```python
from build123d import *

# Parameters (mm, degrees)
SKETCH1_W               = 171.8
SKETCH1_H               = 57.8
MAIN_BODY_DEPTH         = 10
SKETCH2_W               = 163.8
SKETCH2_H               = 49.8
MAIN_CUTOUT_DEPTH       = 8
SKETCH3_W               = 6
SKETCH3_H               = 20
CABLE_PASSTHROUGH_DEPTH = 4
SKETCH9_W               = 168
SKETCH9_H               = 54
LID_CUTOUT_DEPTH        = 2


with BuildPart() as part:
    # Sketch1 → Main_Body (new body)
    with BuildSketch(Plane.XY):
        with Locations((85.9, 28.9)):
            Rectangle(SKETCH1_W, SKETCH1_H)
    extrude(amount=MAIN_BODY_DEPTH)

    # Sketch2 → Main_Cutout (cut)
    with BuildSketch(Plane.XY.offset(10)):
        with Locations((85.9, 28.9)):
            Rectangle(SKETCH2_W, SKETCH2_H)
    extrude(amount=-MAIN_CUTOUT_DEPTH, mode=Mode.SUBTRACT)

    # Sketch3 → Cable_Passthrough (cut)
    with BuildSketch(Plane(origin=(53.8, 57.8, 0), x_dir=(0, 0, 1), z_dir=(0, -1, 0))):
        with Locations((5, -32.1)):
            Rectangle(SKETCH3_W, SKETCH3_H)
    extrude(amount=CABLE_PASSTHROUGH_DEPTH, mode=Mode.SUBTRACT)

    # Sketch9 → Lid_Cutout (cut)
    with BuildSketch(Plane.XY.offset(10)):
        with Locations((85.9, 28.9)):
            Rectangle(SKETCH9_W, SKETCH9_H)
    extrude(amount=-LID_CUTOUT_DEPTH, mode=Mode.SUBTRACT)


solid = part.part
```
Build history of the part. All positions in model axes, mm. A direction names the side the tool comes from. Give positions to 0.01 mm unless a question says otherwise; leave off trailing zeros. Loops run counter-clockwise (first coordinate to the right, second up) from the corner with the lowest first, then second, coordinate; pieces in that order, holes last.
1) 3-axis set-ups, long thin cutter, end or side, ignore diameter. For faces 5 (the face through (85, 29, 0)), 6 (the face through (39, 53.8, 5)), 7 (the face through (75.9, 56, 5)): which of +Z, -Z, +X, -X, +Y, -Y reach the whole face in a straight line?
Values follow:
face 5: -Z, +X, -X, +Y, -Y
face 6: +Z
face 7: +Y
2) Band-saw the part on B-B on y = 17.5. List the corners of the cut face in (x, z).
Values follow:
outline: (0, 0) - (171.8, 0) - (171.8, 10) - (169.9, 10) - (169.9, 8) - (167.8, 8) - (167.8, 2) - (4, 2) - (4, 8) - (1.9, 8) - (1.9, 10) - (0, 10) - close
3) Probe line 1 along X through (y, z) = (37, 8.75); line 2 along Y through (x, z) = (141, 6.5); line 3 along X through (y, z) = (24, 5.5). List the from-to ranges inside material, lowest first.
Values follow:
line 1: x = 0 to 1.9, 169.9 to 171.8
line 2: y = 0 to 4, 53.8 to 57.8
line 3: x = 0 to 4, 167.8 to 171.8
4) Two-plate mould, pull along Y, no slides. Class faces 1 (the face through (167.8, 29, 5)), 2 (the face through (4, 29, 5)), 3 (the face through (84.7, 57.8, 1.6)), 4 (the face through (171.8, 28, 5)): released by +Y, released by -Y, zero draft, split by the parting line, or undercut.
Values follow:
face 1: undercut
face 2: undercut
face 3: released by +Y
face 4: zero draft
5) Band-saw the part on A-A on x = 109. List the corners of the cut face in (y, z), then the cut area to 3 significant figures.
Values follow:
outline: (0, 0) - (57.8, 0) - (57.8, 10) - (55.9, 10) - (55.9, 8) - (53.8, 8) - (53.8, 2) - (4, 2) - (4, 8) - (1.9, 8) - (1.9, 10) - (0, 10) - close
area: 171 mm2
6) Drop a flat-ended pin along its axis: P1, Ø10, axis at x = 131, y = 41.5, coming from the -Z side. Give the stop position or say it passes through.
Values follow:
P1: stops at z = 0
